```python
from build123d import *

# Parameters (mm, degrees)
SKETCH2_W               = 120
SKETCH2_H               = 70
BOSS_EXTRUDE1_DEPTH     = 30
SHELL1_T                = 2
CUT_EXTRUDE1_DEPTH      = 131.969462089
CUT_EXTRUDE1_DEPTH_BACK = 30
SKETCH3_R               = 2.5
BOSS_EXTRUDE2_DEPTH     = 70
CUT_EXTRUDE2_DEPTH      = 79.185676438
CUT_EXTRUDE2_DEPTH_BACK = 79.185676438
BOSS_EXTRUDE3_DEPTH     = 30
SKETCH7_W               = 3.836872944
SKETCH7_H               = 6.434844856
BOSS_EXTRUDE4_DEPTH     = 2
SKETCH8_R               = 2.5
CUT_EXTRUDE5_DEPTH      = 5
BOSS_EXTRUDE5_START     = -30
SKETCH10_W              = 6
SKETCH10_H              = 6
SKETCH10_H_2            = 5.9
BOSS_EXTRUDE5_DEPTH     = 30
SKETCH12_R              = 1.5
CUT_EXTRUDE6_DEPTH      = 15
FILLET2_R               = 1


with BuildPart() as part:
    # Sketch2 → Boss-Extrude1 (new body)
    with BuildSketch(Plane(origin=(0, 0, 0), x_dir=(1, 0, 0), z_dir=(0, 1, 0))):
        Rectangle(SKETCH2_W, SKETCH2_H)
    extrude(amount=BOSS_EXTRUDE1_DEPTH)

    # Shell1
    shell1_openings = [part.faces().sort_by_distance(p)[0] for p in [
        (0, 30, 0),
    ]]
    offset(amount=SHELL1_T, openings=shell1_openings, kind=Kind.INTERSECTION)

    # Sketch3 → Cut-Extrude1 (cut, two sides: drawn at the far end of the back side and taken through both)
    with BuildSketch(Plane(origin=(-60, 0, 0), x_dir=(0, 0, -1), z_dir=(1, 0, 0)).offset(-CUT_EXTRUDE1_DEPTH_BACK)):
        with Locations(Location((-28, 3, 0), (0, 0, 180))):
            Circle(SKETCH3_R)
    extrude(amount=CUT_EXTRUDE1_DEPTH + CUT_EXTRUDE1_DEPTH_BACK, mode=Mode.SUBTRACT)

    # Sketch4 → Boss-Extrude2 (add)
    with BuildSketch(Plane.ZY.offset(-60)):
        with BuildLine():
            ThreePointArc((-12.9, 9.1), (-15.565328291, 2.665328291), (-22, 0))
            Line((-22, 0), (-3.799999988, 0))
            ThreePointArc((-3.799999988, 0), (-10.234671705, 2.665328287), (-12.9, 9.1))
        make_face()
        with BuildLine():
            ThreePointArc((5.3, 9.1), (2.634671713, 2.665328295), (-3.799999988, 0))
            Line((-3.799999988, 0), (14.399999991, 0))
            ThreePointArc((14.399999991, 0), (7.965328288, 2.665328294), (5.3, 9.1))
        make_face()
        with BuildLine():
            ThreePointArc((23.5, 9.1), (20.834671706, 2.665328288), (14.399999991, 0))
            Line((14.399999991, 0), (23.5, 0))
            Line((23.5, 0), (23.5, 9.1))
        make_face()
        with BuildLine():
            ThreePointArc((-22, 0), (-28.434671709, 2.665328291), (-31.1, 9.1))
            Line((-31.1, 9.1), (-31.1, 0))
            Line((-31.1, 0), (-22, 0))
        make_face()
    extrude(amount=BOSS_EXTRUDE2_DEPTH)

    # Sketch5 → Cut-Extrude2 (cut, two sides: drawn at the far end of the back side and taken through both)
    with BuildSketch(Plane(origin=(0, 0, 0), x_dir=(1, 0, 0), z_dir=(0, 1, 0)).offset(-CUT_EXTRUDE2_DEPTH_BACK)):
        Polygon((-55.9, 39.544038894), (-55.9, -29.4), (62, -29.4), (62, -41.301551734), (-55.9, -41.301551734), (-67.058664884, -41.301551734), (-67.058664884, 39.544038894), align=None)
    extrude(amount=CUT_EXTRUDE2_DEPTH + CUT_EXTRUDE2_DEPTH_BACK, mode=Mode.SUBTRACT)

    # Sketch6 → Boss-Extrude3 (add)
    with BuildSketch(Plane(origin=(0, 0, 0), x_dir=(1, 0, 0), z_dir=(0, 1, 0))):
        Polygon((-55.9, 35), (-55.9, -29.4), (62, -29.4), (62, -27.4), (-53.9, -27.4), (-53.9, 35), align=None)
    extrude(amount=BOSS_EXTRUDE3_DEPTH)

    # Sketch7 → Boss-Extrude4 (add)
    with BuildSketch(Plane(origin=(62, 0, 0), x_dir=(0, 0, -1), z_dir=(1, 0, 0))):
        with Locations((-26.496817491, 3.217422428)):
            Rectangle(SKETCH7_W, SKETCH7_H)
    extrude(amount=-BOSS_EXTRUDE4_DEPTH)

    # Sketch8 → Cut-Extrude5 (cut)
    with BuildSketch(Plane(origin=(-53.9, 0, 0), x_dir=(0, 0, -1), z_dir=(1, 0, 0))):
        with Locations((28.5, 2.5)):
            Circle(SKETCH8_R)
    extrude(amount=-CUT_EXTRUDE5_DEPTH, mode=Mode.SUBTRACT)

    # Sketch10 → Boss-Extrude5 (add)
    with BuildSketch(Plane(origin=(0, 30, 0), x_dir=(1, 0, 0), z_dir=(0, 1, 0)).offset(BOSS_EXTRUDE5_START)):
        with Locations((-52.9, 34)):
            Rectangle(SKETCH10_W, SKETCH10_H)
        with Locations((-52.9, -26.4)):
            Rectangle(SKETCH10_W, SKETCH10_H)
        with Locations((59, 34.05)):
            Rectangle(SKETCH10_W, SKETCH10_H_2)
        with Locations((59, -26.4)):
            Rectangle(SKETCH10_W, SKETCH10_H)
    extrude(amount=BOSS_EXTRUDE5_DEPTH)

    # Sketch12 → Cut-Extrude6 (cut)
    with BuildSketch(Plane(origin=(0, 30, 0), x_dir=(1, 0, 0), z_dir=(0, 1, 0))):
        with Locations(Location((-52.9, 34, 0), (0, 0, 270))):
            Circle(SKETCH12_R)
        with Locations(Location((59, 34.05, 0), (0, 0, 270))):
            Circle(SKETCH12_R)
        with Locations(Location((59, -26.4, 0), (0, 0, 270))):
            Circle(SKETCH12_R)
        with Locations(Location((-52.9, -26.4, 0), (0, 0, 270))):
            Circle(SKETCH12_R)
    extrude(amount=-CUT_EXTRUDE6_DEPTH, mode=Mode.SUBTRACT)

    # Fillet2
    fillet2_edges = [part.edges().sort_by_distance(p)[0] for p in [
        (-55.9, -2, -3.8),
        (-55.9, 14, -37),
        (62, 14, 29.4),
        (3.05, -2, 29.4),
        (-55.9, 14, 29.4),
        (3.05, -2, -37),
        (62, 14, -37),
        (62, -2, -3.8),
    ]]
    fillet(fillet2_edges, radius=FILLET2_R)


solid = part.part
```
CAD build for the part. Positions are in the model's coordinates, mm. A direction names the side the tool comes from. Round coordinates to 2 decimals unless told otherwise and drop trailing zeros. Loops run counter-clockwise (first coordinate to the right, second up) from the corner with the lowest first, then second, coordinate; pieces in that order, holes last. Notation, with made-up numbers: (-6, -34.75) - (42, -34.75) arc R24 cw to (42, -18.75) - close; hole circle Ø9 at (46, 6). An arc over 180 degrees is marked (long way). Return JSON: item names as keys, results as strings. Group by question number.
Q1. Drill centre lines: line 1 along X through (y, z) = (20.25, 26.4); line 2 along Z through (x, y) = (-27, 3.5); line 3 along X through (y, z) = (19, 9). Where is each one in solid material? Low to high. Write a range as [from, to].
Q2. Band-saw the part on D-D on x = -29. Give the cut face in (y, z), plus the area to 3 significant figures.
Q3. Band-saw the part on B-B on x = 31. Give the cut face in (y, z).
Q4. Tool access for faces 4 (the face through (62, 14, -3)), 5 (the face through (-54.9, 1, -26.5)), 6 (the face through (60.265, 22.605, 27.206)): list every direction of +Z, -Z, +X, -X, +Y, -Y with a clear straight run to the whole face (end or side of a thin tool).
Q5. Two-plate mould, pull along Z, no slides. Class faces 1 (the face through (2, 14, 29.4)), 2 (the face through (-51.413, 22.605, -34.195)), 3 (the face through (2, -2, -4)): +Z half, -Z half, draft (parallel to the pull), parting line (faces both ways), or undercut.
Q6. Flat gauge pin, fed straight in: pin 1 Ø5 at (x, z) = (-27, -15.5) entering from +Y. Where does the tip first touch, or does it go through?
Q7. Band-saw the part on A-A on y = 19. Give the cut face in (x, z).
Q8. Band-saw the part on C-C on z = 2.5. Give the cut face in (x, y).
Solutions:
{
 "1": {"line 1": "x = [-55.9, -54.4], [-51.4, -49.9], [56, 57.5], [60.5, 62]", "line 2": "z = [-37, -35], [27.4, 29.4]", "line 3": "x = [-55.9, -53.9], [60, 62]"},
 "2": {"outline": "(-2, -36) arc R1 ccw to (-1, -37) - (30, -37) - (30, -35) - (0, -35) - (0, 27.4) - (30, 27.4) - (30, 29.4) - (-1, 29.4) arc R1 ccw to (-2, 28.4) - close", "area": "252 mm^2"},
 "3": {"outline": "(-2, -36) arc R1 ccw to (-1, -37) - (30, -37) - (30, -35) - (0, -35) - (0, -31.1) - (9.1, -31.1) arc R9.1 cw to (9.1, -12.9) arc R9.1 cw to (9.1, 5.3) arc R9.1 cw to (9.1, 23.5) - (0, 23.5) - (0, 27.4) - (30, 27.4) - (30, 29.4) - (-1, 29.4) arc R1 ccw to (-2, 28.4) - close"},
 "4": {"face 4": "+Z, -Z, +X, +Y, -Y", "face 5": "-X", "face 6": "+Y"},
 "5": {"face 1": "+Z half", "face 2": "undercut", "face 3": "draft"},
 "6": {"pin 1": "stops at y = 0"},
 "7": {"outline": "(-55.9, -36) arc R1 ccw to (-54.9, -37) - (61, -37) arc R1 ccw to (62, -36) - (62, 28.4) arc R1 ccw to (61, 29.4) - (-54.9, 29.4) arc R1 ccw to (-55.9, 28.4) - close; hole circle Ø3 at (-52.9, -34); hole circle Ø3 at (-52.9, 26.4); hole (-53.9, -31) - (-49.9, -31) - (-49.9, -35) - (56, -35) - (56, -31.1) - (60, -31.1) - (60, 23.4) - (56, 23.4) - (56, 27.4) - (-49.9, 27.4) - (-49.9, 23.4) - (-53.9, 23.4) - close; hole circle Ø3 at (59, -34.05); hole circle Ø3 at (59, 26.4)"},
 "8": {"outline": "(-55.9, -1) arc R1 ccw to (-54.9, -2) - (61, -2) arc R1 ccw to (62, -1) - (62, 30) - (60, 30) - (60, 2.53) - (-10, 2.53) - (-10, 0) - (-53.9, 0) - (-53.9, 30) - (-55.9, 30) - close"}
}
